```python
from build123d import *

# Parameters (mm, degrees)
EXTRUDE_1_DEPTH      = 76
EXTRUDE_1_DEPTH_BACK = 5
SKETCH_2_R           = 1.2
CUT_EXTRUDE_1_DEPTH  = 78.307052917


with BuildPart() as part:
    # ｽｹｯﾁ1 → ﾎﾞｽ - 押し出し1 (new, two sides: drawn at the far end of the back side and taken through both)
    with BuildSketch(Plane.XY.offset(-EXTRUDE_1_DEPTH_BACK)):
        Polygon((-5, 9.67820323), (-1, 2.75), (-1, -2.75), (1, -2.75), (1, 2.75), (-3, 9.67820323), (-3, 11.67820323), (-5, 11.67820323), (-7, 11.67820323), (-7, 9.67820323), align=None)
    extrude(amount=EXTRUDE_1_DEPTH + EXTRUDE_1_DEPTH_BACK)

    # ｽｹｯﾁ2 → ｶｯﾄ - 押し出し1 (cut, through all)
    with BuildSketch(Plane(origin=(1, 0, 0), x_dir=(0, 0, -1), z_dir=(1, 0, 0))):
        with Locations((-59.5, 0)):
            Circle(SKETCH_2_R)
        with Locations((-11.5, 0)):
            Circle(SKETCH_2_R)
    extrude(amount=-CUT_EXTRUDE_1_DEPTH, mode=Mode.SUBTRACT)


solid = part.part
```
The model under review builds one solid part; all positions refer to its coordinate system, in mm. A direction names the side the tool comes from. Round coordinates to 2 decimals unless told otherwise and drop trailing zeros. Loops run counter-clockwise (first coordinate to the right, second up) from the corner with the lowest first, then second, coordinate; pieces in that order, holes last. Notation, with made-up numbers: (11.25, 51) -> (20.25, 51) arc R21 cw to (20.25, 74) -> close; hole circle Ø9 at (80, -25.5). An arc over 180 degrees is marked (long way). Answer as a JSON object with one key per item and string values. Group by question number.
1) For faces 4 (the face through (-1, 0, 35)), 5 (the face through (-3, 11, 35)), 6 (the face through (0.01, -0.46, 58.39)), list the 3-axis set-ups (+Z, -Z, +X, -X, +Y, -Y) from which the entire face can be reached by the end or side of a thin tool; tool diameter is ignored.
2) We need section A-A on z = 59.5. Write out the cut boundary in (x, y), then the cut area to 3 significant figures.
3) We need section D-D on x = -5.75. Write out the cut boundary in (y, z), then the cut area to 3 significant figures.
4) We need section B-B on y = 0. Write out the cut boundary in (x, z), then the cut area to 3 significant figures.
5) We need section C-C on z = 43. Write out the cut boundary in (x, y).
6) Mouldability with a two-part tool opening along Y and no side actions: class faces 1 (the face through (-5, 11.678, 35)), 2 (the face through (-6, 9.678, 35)), 3 (the face through (0.014, 0.36, 10.355)) as released by +Y, released by -Y, zero draft, split by the parting line, or undercut.
7) For pin 1 Ø1.5 at (x, z) = (-5.5, 14) entering from -Y; pin 2 Ø3 at (y, z) = (7.5, 29) entering from -X; pin 3 Ø6 at (y, z) = (-0.5, 25.5) entering from -X; pin 4 Ø3 at (x, y) = (-6, 7) entering from -Z, all flat-tipped, find the tip position at first contact; note any pin that passes through.
8) For line 1 (X direction, y = 0.5, z = 36); line 2 (Y direction, x = -6.5, z = 0.5); line 3 (Y direction, x = 0.1, z = 11.5), list the stretches that pass through material, from the lowest coordinate up. Write a range as [from, to].
Result set:
{
 "1": {"face 4": "+Z, -Z, -X, -Y", "face 5": "+Z, -Z, +X, +Y", "face 6": "+X, -X"},
 "2": {"outline": "(-7, 9.68) -> (-5, 9.68) -> (-1, 2.75) -> (-1, 1.2) -> (1, 1.2) -> (1, 2.75) -> (-3, 9.68) -> (-3, 11.68) -> (-7, 11.68) -> close; (-1, -2.75) -> (1, -2.75) -> (1, -1.2) -> (-1, -1.2) -> close", "area": "28.1 mm²"},
 "3": {"outline": "(9.68, -5) -> (11.68, -5) -> (11.68, 76) -> (9.68, 76) -> close", "area": "162 mm²"},
 "4": {"outline": "(-1, -5) -> (1, -5) -> (1, 10.3) -> (-1, 10.3) -> close; (-1, 12.7) -> (1, 12.7) -> (1, 58.3) -> (-1, 58.3) -> close; (-1, 60.7) -> (1, 60.7) -> (1, 76) -> (-1, 76) -> close", "area": "152 mm²"},
 "5": {"outline": "(-7, 9.68) -> (-5, 9.68) -> (-1, 2.75) -> (-1, -2.75) -> (1, -2.75) -> (1, 2.75) -> (-3, 9.68) -> (-3, 11.68) -> (-7, 11.68) -> close"},
 "6": {"face 1": "released by +Y", "face 2": "released by -Y", "face 3": "undercut"},
 "7": {"pin 1": "y = 9.25", "pin 2": "x = -4.61", "pin 3": "x = -1", "pin 4": "through"},
 "8": {"line 1": "[-1, 1]", "line 2": "[9.68, 11.68]", "line 3": "[-2.75, -1.2], [1.2, 4.31]"}
}
